Geometry check sheet. Reference: the model listing, model coordinates, mm. Face numbers are marked on the shaded views. A direction names the side the tool comes from. Give positions to 0.01 mm unless a question says otherwise; leave off trailing zeros. Write each loop counter-clockwise with the first axis right and the second up, starting at its lowest first coordinate (ties: lowest second). Pieces come first, ordered by that corner, then holes. Notation, with made-up numbers: (-16, 69.5) -> (23, 69.5) arc R13 ccw to (23, 77.5) -> close; hole circle Ø6 at (54.25, 19.5). An arc over 180 degrees is marked (long way). Use a Markdown table: item, result. Add a question column.
Autodesk Inventor part; units mm, degrees
ref_plane "YZ Plane" through (0, 0, 0) normal (1, 0, 0) x (0, 1, 0)
ref_plane "XZ Plane" through (0, 0, 0) normal (0, 1, 0) x (-1, 0, 0)
ref_plane "XY Plane" through (0, 0, 0) normal (0, 0, 1) x (1, 0, 0)
sketch "Sketch1" plane through (0, 0, 0) normal (1, 0, 0) x (0, 1, 0)
  line L0 (0, 0) -> (16.51, 0)
  line L1 (16.51, 0) -> (16.51, -63.5)
  line L2 (16.51, -63.5) -> (0, -63.5)
  line L3 (0, -63.5) -> (0, 0)
  circle A0 centre (4.445, -7.62) radius 2.4329
  circle A1 centre (4.445, -15.6185) radius 2.4329
  circle A2 centre (4.445, -23.6169) radius 2.4329
  circle A3 centre (4.445, -31.6154) radius 2.4329
  circle A4 centre (4.445, -39.6138) radius 2.4329
  circle A5 centre (4.445, -47.6123) radius 2.4329
  circle A6 centre (4.445, -55.6108) radius 2.4329
  dimension "d0" = 63.5
  dimension "d1" = 16.51
  dimension "d6" = 7.9985
  dimension "d11" = 7.62
extrude "Extrusion1" add sketch "Sketch1" along normal blind 4.7625
sketch "Sketch2" plane through (4.7625, 0, 0) normal (1, 0, 0) x (0, 0, -1)
  line L0 (63.5, 16.51) -> (0, 16.51)
  line L1 (63.5, 0) -> (63.5, 16.51)
  line L2 (0, 16.51) -> (63.5, 16.51)
  line L3 (63.5, 16.51) -> (63.5, 13.208)
  line L4 (63.5, 13.208) -> (0, 13.208)
  line L5 (0, 13.208) -> (0, 16.51)
  point P0 (0, 0)
  dimension "d14" = 3.302
extrude "Extrusion2" add sketch "Sketch2" along normal blind 1.016
sketch "Sketch3" plane through (0, 0, 0) normal (0, 0, 1) x (1, 0, 0)
  line L0 (5.7785, 16.51) -> (5.7785, 13.208)
  arc A0 (15.8804, 9.6157) -> (23.749, 16.51) centre (23.749, 8.5725) ccw
  line L1 (0, 16.51) -> (0, 0)
  line L2 (5.7785, 16.51) -> (23.749, 16.51)
  line L3 (4.7625, 13.208) -> (5.7785, 13.208)
  line L4 (5.7785, 13.208) -> (12.7329, 13.208)
  arc A1 (15.8804, 9.6157) -> (12.7329, 13.208) centre (12.7329, 10.033) ccw
  point P0 (17.3057, 13.208)
  point P1 (9.5258, 13.208)
  dimension "d17" = 23.749
  dimension "d18" = 15.875
  dimension "d19" = 3.175
extrude "Extrusion3" add sketch "Sketch3" against normal blind 63.5
sketch "Sketch4" plane through (0, 16.51, 0) normal (0, 1, 0) x (1, 0, 0)
  line L0 (31.6865, 0) -> (31.6865, 63.5)
  line L1 (31.6865, 0) -> (31.6865, 83.2403)
  point P0 (0, 0)
properties part number "knuckle plate"
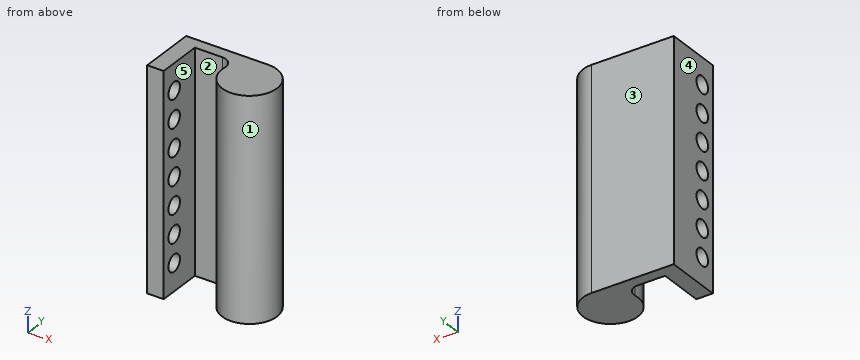
1) Sectioned sample at C-C, the plane z = -59. Enter the section's corners in (x, y), and give its area (3 significant figures).
2) Sectioned sample at D-D, the plane x = 6. Enter the section's corners in (y, z), and give its area (3 significant figures).
3) Draft check along X on the marked faces 3, 4 and 5. Enter one of: +X half, -X half, draft (parallel to the pull), parting line (faces both ways), or undercut.
4) Gauge pin test, flat ends, axial feed: P1, Ø1.5, axis at y = 7, z = -36.5, coming from the +X side; P2, Ø4, axis at y = 12.5, z = -38.5, coming from the +X side; P3, Ø4, axis at x = 3.5, y = 9.5, coming from the +Z side; P4, Ø1, axis at y = 15, z = -27.5, coming from the +X side. Record the tip position at first contact, or that the pin passes through.
5) Sectioned sample at A-A, the plane y = 11.25. Enter the section's corners in (x, z).
6) Material ranges on probe 1 along Y at (x, z) = (2.5, -7.5); probe 2 along X at (y, z) = (9, -47.5); probe 3 along Y at (x, z) = (10, -31.5), recorded low to high. Write a range as [from, to].
7) Sectioned sample at B-B, the plane z = -7.62. Enter the section's corners in (x, y), and give its area (3 significant figures).
8) Tool access check on the marked faces 1 and 2. Record the directions out of +Z, -Z, +X, -X, +Y, -Y that give a thin tool (end or side, any length) a straight path to the whole face; none if there is none.
Check values:
| question | item | result |
|---|---|---|
| 1 | outline | (0, 0) -> (4.76, 0) -> (4.76, 13.21) -> (12.73, 13.21) arc R3.17 cw to (15.88, 9.62) arc R7.94 ccw (long way) to (23.75, 16.51) -> (0, 16.51) -> close |
| 1 | area | 328 mm² |
| 2 | outline | (13.21, -63.5) -> (16.51, -63.5) -> (16.51, 0) -> (13.21, 0) -> close |
| 2 | area | 210 mm² |
| 3 | face 3 | draft |
| 3 | face 4 | -X half |
| 3 | face 5 | undercut |
| 4 | P1 | x = 31.64 |
| 4 | P2 | x = 31.45 |
| 4 | P3 | z = 0 |
| 4 | P4 | x = 29.03 |
| 5 | outline | (0, -63.5) -> (4.76, -63.5) -> (4.76, 0) -> (0, 0) -> close; (15.67, -63.5) -> (31.22, -63.5) -> (31.22, 0) -> (15.67, 0) -> close |
| 6 | probe 1 | [0, 2.02], [6.87, 16.51] |
| 6 | probe 2 | [0, 4.76], [15.82, 31.67] |
| 6 | probe 3 | [13.21, 16.51] |
| 7 | outline | (0, 0) -> (4.76, 0) -> (4.76, 2.01) -> (0, 2.01) -> close; (0, 6.88) -> (4.76, 6.88) -> (4.76, 13.21) -> (12.73, 13.21) arc R3.17 cw to (15.88, 9.62) arc R7.94 ccw (long way) to (23.75, 16.51) -> (0, 16.51) -> close |
| 7 | area | 305 mm² |
| 8 | face 1 | +Z, -Z |
| 8 | face 2 | +Z, -Z, -Y |
